Read the model definition and answer for the solid it produces. Units are mm, in the model's axes. A direction names the side the tool comes from. Round coordinates to 2 decimals unless told otherwise and drop trailing zeros. Loops run counter-clockwise (first coordinate to the right, second up) from the corner with the lowest first, then second, coordinate; pieces in that order, holes last. Notation, with made-up numbers: (8, 39.5) - (60, 39.5) arc R21 cw to (60, 46.5) - close; hole circle Ø3 at (28.25, 39.25). An arc over 180 degrees is marked (long way). Answer as CSV lines item,"result".
```python
from build123d import *

# Parameters (mm, degrees)
F0_R     = 1.75
F0_R_2   = 1.625
F1_DEPTH = 11.05


with BuildPart() as f1:
    # F0 (on Front) → F1 (new body)
    with BuildSketch(Plane.XZ):
        with BuildLine():
            Line((-7.5, -3.5), (-0.620029, -4.45708))
            ThreePointArc((-0.620029, -4.45708), (-0.310756, -4.489257), (0, -4.5))
            Line((0, -4.5), (11.839124, -4.5))
            ThreePointArc((11.839124, -4.5), (24.369894, -6.368848), (36.860822, -4.25))
            Line((36.860822, -4.25), (47.5, -4.25))
            ThreePointArc((47.5, -4.25), (49.476882, -3.762239), (51, -2.410913))
            Line((51, -2.410913), (51, 2.410913))
            ThreePointArc((51, 2.410913), (48.261956, 4.181139), (45.075467, 3.490578))
            ThreePointArc((45.075467, 3.490578), (23.808304, -3.120513), (2.598914, 3.673642))
            ThreePointArc((2.598914, 3.673642), (1.363564, 4.288437), (0, 4.5))
            Line((0, 4.5), (-7.5, 4.5))
            Line((-7.5, 4.5), (-7.5, -3.5))
        make_face()
        Circle(F0_R, mode=Mode.SUBTRACT)
        with Locations((47.5, 0)):
            Circle(F0_R_2, mode=Mode.SUBTRACT)
    extrude(amount=F1_DEPTH)


solid = f1.part
```
1) A cutting plane is placed at D-D, the plane x = 42.5. Determine the outline of the cut face in (y, z), plus the area to 3 significant figures.
Entries:
outline,"(-11.05, -4.25) - (0, -4.25) - (0, 1.85) - (-11.05, 1.85) - close"
area,"67.5 mm^2"
2) Find the intervals of material crossed by line 1 (Z direction, x = 47.5, y = -3.75) (3 decimals); line 2 (X direction, y = -3.5, z = 0.75); line 3 (X direction, y = -8.75, z = 0.5), in increasing order.
Entries:
line 1,"z = -4.25 to -1.625, 1.625 to 4.25"
line 2,"x = -7.5 to -1.58, 1.58 to 7.49, 40.44 to 46.06, 48.94 to 51"
line 3,"x = -7.5 to -1.68, 1.68 to 8, 39.93 to 45.95, 49.05 to 51"
3) A tool of negligible diameter and unlimited length cuts with its end or side. For faces 4 (the face through (42, -5, -4.25)), 5 (the face through (51, -5, 0)), 6 (the face through (6, -5, -4.5)), 7 (the face through (1.382, -5.448, 4.283)), from which of +Z, -Z, +X, -X, +Y, -Y can it reach the whole face along a straight path? Write none if from no direction.
Entries:
face 4,"-Z, +X, +Y, -Y"
face 5,"+Z, -Z, +X, +Y, -Y"
face 6,"-Z, -X, +Y, -Y"
face 7,"+Z, +Y, -Y"
4) A cutting plane is placed at C-C, the plane y = -7.5. Determine the outline of the cut face in (x, z) (3 decimals), plus the area to 3 significant figures.
Entries:
outline,"(-7.5, -3.5) - (-0.62, -4.457) arc R4.5 ccw to (0, -4.5) - (11.839, -4.5) arc R40.25 ccw to (36.861, -4.25) - (47.5, -4.25) arc R4.25 ccw to (51, -2.411) - (51, 2.411) arc R4.25 ccw to (45.075, 3.491) arc R37 cw to (2.599, 3.674) arc R4.5 ccw to (0, 4.5) - (-7.5, 4.5) - close; hole circle Ø3.5 at (0, 0); hole circle Ø3.25 at (47.5, 0)"
area,"293 mm^2"
5) Each of these flat-tipped pins is pushed along its axis until it touches: P1, Ø1.9, axis at x = 47.5, z = 0, coming from the +Y side; P2, Ø5.5, axis at x = 5.5, y = -5.5, coming from the -Z side; P3, Ø5, axis at x = 13.5, y = -6.5, coming from the -Z side; P4, Ø3, axis at x = 43.5, y = -5.5, coming from the -Z side. Where does it stop, or does it pass through?
Entries:
P1,"passes through"
P2,"stops at z = -4.5"
P3,"stops at z = -5.57"
P4,"stops at z = -4.25"
6) A cutting plane is placed at A-A, the plane x = 0.5. Determine the outline of the cut face in (y, z), plus the area to 3 significant figures.
Entries:
outline,"(-11.05, -4.5) - (0, -4.5) - (0, -1.68) - (-11.05, -1.68) - close; (-11.05, 1.68) - (0, 1.68) - (0, 4.47) - (-11.05, 4.47) - close"
area,"62.1 mm^2"
7) A cutting plane is placed at B-B, the plane z = 0. Determine the outline of the cut face in (x, y) (3 decimals), plus the area to 3 significant figures.
Entries:
outline,"(-7.5, -11.05) - (-1.75, -11.05) - (-1.75, 0) - (-7.5, 0) - close; (1.75, -11.05) - (9.095, -11.05) - (9.095, 0) - (1.75, 0) - close; (38.841, -11.05) - (45.875, -11.05) - (45.875, 0) - (38.841, 0) - close; (49.125, -11.05) - (51, -11.05) - (51, 0) - (49.125, 0) - close"
area,"243 mm^2"
8) The mould has two halves that part along X. Classify faces 1 (the face through (-4.11, -5.45, -3.97)), 2 (the face through (24.19, -5.45, -6.37)), 3 (the face through (24.13, -5.45, -3.12)): pulls with the +X half, pulls with the -X half, needs draft (parallel to the pull), parting line crosses it, or undercut.
Entries:
face 1,"pulls with the -X half"
face 2,"parting line crosses it"
face 3,"undercut"
